```python
from build123d import *

# Parameters (mm, degrees)
BOSS_EXTRUDE6_DEPTH                          = 60
CUT_EXTRUDE3_DEPTH                           = 1
CUT_EXTRUDE3_DEPTH_BACK                      = 50
BOSS_EXTRUDE9_DEPTH                          = 50
CUT_EXTRUDE7_DEPTH                           = 25
CBORE_FOR_M8_HEX_HEAD_CAP_SCREW3_D           = 10
CBORE_FOR_M8_HEX_HEAD_CAP_SCREW3_DEPTH       = 10
CBORE_FOR_M8_HEX_HEAD_CAP_SCREW3_CBORE_D     = 15
CBORE_FOR_M8_HEX_HEAD_CAP_SCREW3_CBORE_DEPTH = 5
CBORE_FOR_M8_HEX_HEAD_CAP_SCREW3_TIP         = 3.004303095
CUT_EXTRUDE8_DEPTH                           = 60
SKETCH29_R                                   = 12.5
BOSS_EXTRUDE10_DEPTH                         = 15
SKETCH2_10_R                                 = 12.5
BOSS_EXTRUDE11_DEPTH                         = 15
BOSS_EXTRUDE8_DEPTH                          = 50
CUT_EXTRUDE5_DEPTH                           = 25
CUT_EXTRUDE6_DEPTH                           = 60


with BuildPart() as part:
    # Sketch2 → Boss-Extrude6 (new body)
    with BuildSketch(Plane.XY):
        with BuildLine():
            Line((44, 20), (14.028925254, -12.813635558))
            ThreePointArc((14.028925254, -12.813635558), (0, -19), (-14.028925254, -12.813635558))
            Line((-14.028925254, -12.813635558), (-44, 20))
            Line((-44, 20), (-44, 105))
            Line((-44, 105), (-25, 105))
            ThreePointArc((-25, 105), (-20.757359313, 106.757359313), (-19, 111))
            ThreePointArc((-19, 111), (0, 130), (19, 111))
            ThreePointArc((19, 111), (20.757359313, 106.757359313), (25, 105))
            Line((25, 105), (44, 105))
            Line((44, 105), (44, 20))
        make_face()
    extrude(amount=BOSS_EXTRUDE6_DEPTH)

    # Sketch5 → Cut-Extrude3 (cut, two sides)
    with BuildSketch(Plane.XY.offset(60)) as cut_extrude3_sk:
        with BuildLine():
            Line((14.028925254, -12.813635558), (44, 20))
            Line((44, 20), (44, 92))
            Line((44, 92), (22, 92))
            ThreePointArc((22, 92), (19.878679656, 91.121320344), (19, 89))
            Line((19, 89), (-19, 89))
            ThreePointArc((-19, 89), (-19.878679656, 91.121320344), (-22, 92))
            Line((-22, 92), (-44, 92))
            Line((-44, 92), (-44, 20))
            Line((-44, 20), (-14.028925254, -12.813635558))
            ThreePointArc((-14.028925254, -12.813635558), (0, -19), (14.028925254, -12.813635558))
        make_face()
    extrude(amount=CUT_EXTRUDE3_DEPTH, mode=Mode.SUBTRACT)
    extrude(cut_extrude3_sk.sketch, amount=-CUT_EXTRUDE3_DEPTH_BACK, mode=Mode.SUBTRACT)

    # Sketch5<11> → Boss-Extrude9 (add)
    with BuildSketch(Plane.XY.offset(60)):
        with BuildLine():
            ThreePointArc((-6, 83), (-7.757359313, 87.242640687), (-12, 89))
            Line((-12, 89), (12, 89))
            ThreePointArc((12, 89), (7.757359313, 87.242640687), (6, 83))
            Line((6, 83), (6, 30))
            ThreePointArc((6, 30), (7.757359313, 25.757359313), (12, 24))
            Line((12, 24), (9.5, 24))
            Line((9.5, 24), (-9.5, 24))
            Line((-9.5, 24), (-12, 24))
            ThreePointArc((-12, 24), (-7.757359313, 25.757359313), (-6, 30))
            Line((-6, 30), (-6, 83))
        make_face()
    extrude(amount=-BOSS_EXTRUDE9_DEPTH)

    # Sketch25 → Cut-Extrude7 (cut, symmetric)
    with BuildSketch(Plane(origin=(6, 0, 0), x_dir=(0, 0, -1), z_dir=(1, 0, 0))):
        Polygon((-60, 89), (-10, 24), (-60, 24), (-60, 30), (-60, 83), align=None)
    extrude(amount=CUT_EXTRUDE7_DEPTH, both=True, mode=Mode.SUBTRACT)

    # CBORE for M8 Hex Head Cap Screw3
    with Locations(Plane(origin=(-25, 55, 10), x_dir=(1, 0, 0), z_dir=(0, 0, 1))):
        with Locations((0, 0), (50, 0)):
            CounterBoreHole(CBORE_FOR_M8_HEX_HEAD_CAP_SCREW3_D / 2, CBORE_FOR_M8_HEX_HEAD_CAP_SCREW3_CBORE_D / 2, CBORE_FOR_M8_HEX_HEAD_CAP_SCREW3_CBORE_DEPTH, depth=CBORE_FOR_M8_HEX_HEAD_CAP_SCREW3_DEPTH)
            with Locations((0, 0, -(CBORE_FOR_M8_HEX_HEAD_CAP_SCREW3_DEPTH + CBORE_FOR_M8_HEX_HEAD_CAP_SCREW3_TIP / 2))):  # 118° drill point
                Cone(0, CBORE_FOR_M8_HEX_HEAD_CAP_SCREW3_D / 2, CBORE_FOR_M8_HEX_HEAD_CAP_SCREW3_TIP, mode=Mode.SUBTRACT)

    # Sketch28 → Cut-Extrude8 (cut)
    with BuildSketch(Plane.XY.offset(60)):
        with BuildLine():
            ThreePointArc((0, 101.5), (9.5, 111), (0, 120.5))
            ThreePointArc((0, 120.5), (-9.5, 111), (0, 101.5))
        make_face()
    extrude(amount=-CUT_EXTRUDE8_DEPTH, mode=Mode.SUBTRACT)

    # Sketch29 → Boss-Extrude10 (add)
    with BuildSketch(Plane.XY.offset(10)):
        Circle(SKETCH29_R)
    extrude(amount=BOSS_EXTRUDE10_DEPTH)

    # Sketch2<10> → Boss-Extrude11 (add)
    with BuildSketch(Plane.XY):
        Circle(SKETCH2_10_R)
    extrude(amount=-BOSS_EXTRUDE11_DEPTH)

    # Sketch5<9> → Boss-Extrude8 (add)
    with BuildSketch(Plane.XY.offset(60)):
        with BuildLine():
            ThreePointArc((-6, 83), (-7.757359313, 87.242640687), (-12, 89))
            Line((-12, 89), (12, 89))
            ThreePointArc((12, 89), (7.757359313, 87.242640687), (6, 83))
            Line((6, 83), (6, 30))
            ThreePointArc((6, 30), (7.757359313, 25.757359313), (12, 24))
            Line((12, 24), (9.5, 24))
            Line((9.5, 24), (-9.5, 24))
            Line((-9.5, 24), (-12, 24))
            ThreePointArc((-12, 24), (-7.757359313, 25.757359313), (-6, 30))
            Line((-6, 30), (-6, 83))
        make_face()
    extrude(amount=-BOSS_EXTRUDE8_DEPTH)

    # Sketch11 → Cut-Extrude5 (cut, symmetric)
    with BuildSketch(Plane(origin=(6, 0, 0), x_dir=(0, 0, -1), z_dir=(1, 0, 0))):
        Polygon((-10, 24), (-60, 89), (-60, 83), (-60, 30), (-60, 24), align=None)
    extrude(amount=CUT_EXTRUDE5_DEPTH, both=True, mode=Mode.SUBTRACT)

    # Sketch34 → CSK for M8 Flat Head Machine Screw2 (revolve, cut)
    with BuildSketch(Plane(origin=(0, 0, 25), x_dir=(0, -1, 0), z_dir=(1, 0, 0))):
        Polygon((0, 0), (0, 42.403442476), (4, 40), (4, 6), (10, 0), align=None)
    revolve(axis=Axis((0, 0, 31.35), (0, 0, -1)), mode=Mode.SUBTRACT)

    # Sketch13 → Cut-Extrude6 (cut)
    with BuildSketch(Plane.XY.offset(60)):
        with BuildLine():
            ThreePointArc((0, 101.5), (9.5, 111), (0, 120.5))
            ThreePointArc((0, 120.5), (-9.5, 111), (0, 101.5))
        make_face()
    extrude(amount=-CUT_EXTRUDE6_DEPTH, mode=Mode.SUBTRACT)


solid = part.part
```
The listing builds one solid part. Answer for the finished solid, in the listing's coordinates (mm). A direction names the side the tool comes from. Coordinates: 2 decimals unless noted, no trailing zeros. Write each loop counter-clockwise with the first axis right and the second up, starting at its lowest first coordinate (ties: lowest second). Pieces come first, ordered by that corner, then holes. Notation, with made-up numbers: (45.25, 42) - (85.25, 42) arc R22 ccw to (85.25, 55) - close; hole circle Ø8 at (71, 63.5). An arc over 180 degrees is marked (long way). One line per item, written item: value.
1) A tool of negligible diameter and unlimited length cuts with its end or side. For faces 1 (the cylindrical face through (19.9, 91.14, 35.35)), 2 (the flat face through (-35, 105, 30)), 3 (the cylindrical face through (-19.86, 91.1, 35.35)), from which of +Z, -Z, +X, -X, +Y, -Y can it reach the whole face along a straight path? Write none if from no direction.
Geometry check:
face 1: +Z, +X, -Y
face 2: +Z, -Z, -X, +Y
face 3: +Z, -X, -Y
2) Find section C-C (x = -27). Give the vertices of the cut face in (y, z).
Geometry check:
outline: (1.39, 0) - (50.42, 0) - (50.42, 5) - (47.77, 5) - (47.77, 10) - (1.39, 10) - close; (59.58, 0) - (105, 0) - (105, 60) - (92, 60) - (92, 10) - (62.23, 10) - (62.23, 5) - (59.58, 5) - close
3) Each of these flat-tipped pins is pushed along its axis until it touches: pin 1 Ø5.5 at (x, z) = (-38.5, 33.5) entering from +Y; pin 2 Ø12 at (x, y) = (-1.5, 49.5) entering from -Z; pin 3 Ø4.5 at (x, y) = (26.5, 58.5) entering from +Z. Where does it stop, or does it pass through?
Geometry check:
pin 1: stops at y = 105
pin 2: stops at z = 0
pin 3: stops at z = 5
4) Consider line 1 along Z through (x, y) = (4.5, 20); line 2 along X through (y, z) = (116, 51); line 3 along Y through (x, z) = (30, 7). Determine where each line is inside the solid, lowest interval first. Write a range as from..to.
Geometry check:
line 1: z = 0..10
line 2: x = -18.33..-8.08, 8.08..18.33
line 3: y = 4.67..49.41, 60.59..105
5) Find section D-D (y = 114). Give the vertices of the cut face in (x, z), and give its area (3 significant figures).
Geometry check:
outline: (-18.76, 0) - (-9.01, 0) - (-9.01, 60) - (-18.76, 60) - close; (9.01, 0) - (18.76, 0) - (18.76, 60) - (9.01, 60) - close
area: 1,170 mm2
6) For a pull along Y with two mould halves and no side action, classify faces 4 (the flat face through (34, 105, 30)), 5 (the cylindrical face through (11.923, 3.755, -7.395)), 6 (the cylindrical face through (-6.59, 27.405, 11.314)), 7 (the cylindrical face through (-7.711, 87.196, 35.35)) as pulls with the +Y half, pulls with the -Y half, needs draft (parallel to the pull), parting line crosses it, or undercut.
Geometry check:
face 4: pulls with the +Y half
face 5: parting line crosses it
face 6: undercut
face 7: undercut
7) Find section B-B (z = 30). Give the vertices of the cut face in (x, y).
Geometry check:
outline: (-44, 92) - (-22, 92) arc R3 cw to (-19, 89) - (-12, 89) arc R6 cw to (-6, 83) - (-6, 50) - (6, 50) - (6, 83) arc R6 cw to (12, 89) - (19, 89) arc R3 cw to (22, 92) - (44, 92) - (44, 105) - (25, 105) arc R6 cw to (19, 111) arc R19 ccw to (-19, 111) arc R6 cw to (-25, 105) - (-44, 105) - close; hole circle Ø19 at (0, 111)
8) Find section A-A (y = 52.5). Give the vertices of the cut face in (x, z), and give its area (3 significant figures).
Geometry check:
outline: (-44, 0) - (-29.33, 0) - (-29.33, 5) - (-32.07, 5) - (-32.07, 10) - (-44, 10) - close; (-20.67, 0) - (20.67, 0) - (20.67, 5) - (17.93, 5) - (17.93, 10) - (6, 10) - (6, 31.92) - (-6, 31.92) - (-6, 10) - (-17.93, 10) - (-17.93, 5) - (-20.67, 5) - close; (29.33, 0) - (44, 0) - (44, 10) - (32.07, 10) - (32.07, 5) - (29.33, 5) - close
area: 915 mm2
